Could you check a few things on this model? Use its own coordinates, in mm. A direction names the side the tool comes from. Round coordinates to 2 decimals unless told otherwise and drop trailing zeros. Loops run counter-clockwise (first coordinate to the right, second up) from the corner with the lowest first, then second, coordinate; pieces in that order, holes last. Notation, with made-up numbers: (-30, 84) -> (-21, 84) arc R11 cw to (-21, 103) -> close; hole circle Ø1 at (30, 45.5). An arc over 180 degrees is marked (long way). One line per item, written item: value.
from build123d import *

# Parameters (mm, degrees)
F0_R      = 50.8
F1_DEPTH  = 6.35
F2_W      = 12.7
F2_H      = 12.7
F3_DEPTH  = 12.7
F4_R      = 6.34999
F5_R      = 3.175
F6_DEPTH  = 57.151
F7_R      = 3.175
F7_R_2    = 19.05
F8_DEPTH  = 6.351
F10_DEPTH = 6.351


# Not quite as in the source:
# - a fillet or chamfer is up to 0.001 mm smaller than in the source, because OpenCascade refuses the exact size


with BuildPart() as f1:
    # F0 (on Front) → F1 (new body)
    with BuildSketch(Plane.XZ):
        Circle(F0_R)
    extrude(amount=F1_DEPTH)

    # F2 (on face) → F3 (join)
    with BuildSketch(Plane.XZ.offset(6.35)):
        with Locations((0, 38.1)):
            Rectangle(F2_W, F2_H)
    extrude(amount=F3_DEPTH)

    # F4 (radius 6.35 in the source; OpenCascade refuses exactly that, so slightly less here)
    f4_edges = [f1.edges().sort_by_distance(p)[0] for p in [
        (0, -19.05, 31.75),
        (0, -19.05, 44.45),
    ]]
    fillet(f4_edges, radius=F4_R)

    # F5 (on face) → F6 (cut, through all)
    with BuildSketch(Plane(origin=(-6.35, 0, 0), x_dir=(0, -1, 0), z_dir=(-1, 0, 0))):
        with Locations((12.7, 38.1)):
            Circle(F5_R)
    extrude(amount=-F6_DEPTH, mode=Mode.SUBTRACT)

    # F7 (on face) → F8 (cut, through all)
    with BuildSketch(Plane.XZ.offset(6.35)):
        with Locations((-38.1, 0)):
            Circle(F7_R)
        with Locations((38.1, 0)):
            Circle(F7_R)
        Circle(F7_R_2)
    extrude(amount=-F8_DEPTH, mode=Mode.SUBTRACT)

    # F9 (on face) → F10 (cut, through all)
    with BuildSketch(Plane.XZ.offset(6.35)):
        with BuildLine():
            Line((-24.5934442484, 44.45), (6.35, 44.45))
            Line((6.35, 44.45), (24.5934442484, 44.45))
            ThreePointArc((24.5934442484, 44.45), (0, 50.8), (-24.5934442484, 44.45))
        make_face()
    extrude(amount=-F10_DEPTH, mode=Mode.SUBTRACT)


solid = f1.part
(1) If we section it at B-B, the plane z = 0: Please give me the cut outline in (x, y) (3 decimals).
Recorded:
outline: (-50.8, -6.35) -> (-41.275, -6.35) -> (-41.275, 0) -> (-50.8, 0) -> close; (-34.925, -6.35) -> (-19.05, -6.35) -> (-19.05, 0) -> (-34.925, 0) -> close; (19.05, -6.35) -> (34.925, -6.35) -> (34.925, 0) -> (19.05, 0) -> close; (41.275, -6.35) -> (50.8, -6.35) -> (50.8, 0) -> (41.275, 0) -> close
(2) I'm going to push flat-ended pins straight in: pin 1 Ø1.9 at (x, y) = (2, -11) entering from -Z; pin 2 Ø5 at (x, z) = (38.1, 0) entering from -Y; pin 3 Ø12 at (x, z) = (-28.5, 28.5) entering from -Y; pin 4 Ø4 at (y, z) = (-11, 39) entering from -X. Where does each tip first touch, or does it pass through?
Recorded:
pin 1: z = 31.75
pin 2: through
pin 3: y = -6.35
pin 4: x = -6.35
(3) If we section it at D-D, the plane y = -2.75: Please give me the cut outline in (x, z) (3 decimals).
Recorded:
outline: (-24.593, 44.45) arc R50.8 ccw (long way) to (24.593, 44.45) -> close; hole circle Ø6.35 at (-38.1, 0); hole circle Ø38.1 at (0, 0); hole circle Ø6.35 at (38.1, 0)
(4) If we section it at C-C, the plane z = -16: Please give me the cut outline in (x, y), then the cut area to 3 significant figures.
Recorded:
outline: (-48.21, -6.35) -> (-10.34, -6.35) -> (-10.34, 0) -> (-48.21, 0) -> close; (10.34, -6.35) -> (48.21, -6.35) -> (48.21, 0) -> (10.34, 0) -> close
area: 481 mm²
(5) If I drill on L1, parallel to Z at x = -3.5, y = -12.7 (3 decimals); L2, parallel to Z at x = 0, y = -1.25; L3, parallel to Y at x = -30, z = 26.5, over which ranges is the centre line in solid material (lowest first)?
Recorded:
L1: 31.75 to 34.925, 41.275 to 44.45
L2: -50.8 to -19.05, 19.05 to 44.45
L3: -6.35 to 0
(6) If we section it at A-A, the plane x = 0: Give the number of separate pieces and of enclosed holes in the cut face, then the cut area to 3 significant figures.
Recorded:
separate pieces: 2
enclosed holes: 1
area: 475 mm²
(7) Thinking about a two-plate mould opening in Z: for faces 1 (the face through (-0.09, -10.18, 36.17)), 2 (the face through (0.09, -17.14, 33.56)), 3 (the face through (-1, -6.35, -24)), which applies, released by +Z, released by -Z, zero draft, split by the parting line, or undercut?
Recorded:
face 1: undercut
face 2: released by -Z
face 3: zero draft
(8) For faces 4 (the face through (-6.35, -11, 35)), 5 (the face through (0.09, -17.14, 42.64)), 6 (the face through (0, -9, 31.75)), 7 (the face through (34.93, -3.22, 0.14)), 8 (the face through (6.35, -11, 35)), which set-ups out of +Z, -Z, +X, -X, +Y, -Y let a thin tool reach every point of the face, with its end or its side?
Recorded:
face 4: +Z, -Z, -X, -Y
face 5: +Z, +X, -X, -Y
face 6: -Z, +X, -X, -Y
face 7: +Y, -Y
face 8: +Z, -Z, +X, -Y
